from build123d import *

# Parameters (mm, degrees)
SKETCH_4_W      = 37
SKETCH_4_H      = 57
EXTRUDE_1_DEPTH = 2
SKETCH_5_W      = 5.285714285
SKETCH_5_H      = 2
SKETCH_5_W_2    = 5.285714286
EXTRUDE_2_DEPTH = 2
EXTRUDE_START   = -57
SKETCH_5_3_W    = 5.285714285
SKETCH_5_3_H    = 2
SKETCH_5_3_W_2  = 5.285714286
EXTRUDE_3_DEPTH = 2
SKETCH_6_W      = 8.142857143
SKETCH_6_H      = 2
SKETCH_6_W_2    = 8.142857142
EXTRUDE_4_DEPTH = 2
EXTRUDE_START_2 = -37
SKETCH_6_2_W    = 8.142857143
SKETCH_6_2_H    = 2
SKETCH_6_2_W_2  = 8.142857142
EXTRUDE_5_DEPTH = 2


with BuildPart() as part:
    # 草图4 → 凸台-拉伸1 (new body)
    with BuildSketch(Plane(origin=(0, 0, 0), x_dir=(1, 0, 0), z_dir=(0, 1, 0))):
        Rectangle(SKETCH_4_W, SKETCH_4_H)
    extrude(amount=EXTRUDE_1_DEPTH)

    # 草图5 → 凸台-拉伸2 (add)
    with BuildSketch(Plane.XY.offset(28.5)):
        with Locations((10.571428572, 1)):
            Rectangle(SKETCH_5_W, SKETCH_5_H)
        with Locations((0, 1)):
            Rectangle(SKETCH_5_W_2, SKETCH_5_H)
        with Locations((-10.571428572, 1)):
            Rectangle(SKETCH_5_W, SKETCH_5_H)
    extrude(amount=EXTRUDE_2_DEPTH)

    # 草图5<3> → 凸台-拉伸3 (add)
    with BuildSketch(Plane.XY.offset(28.5).offset(EXTRUDE_START)):
        with Locations((10.571428572, 1)):
            Rectangle(SKETCH_5_3_W, SKETCH_5_3_H)
        with Locations((0, 1)):
            Rectangle(SKETCH_5_3_W_2, SKETCH_5_3_H)
        with Locations((-10.571428572, 1)):
            Rectangle(SKETCH_5_3_W, SKETCH_5_3_H)
    extrude(amount=-EXTRUDE_3_DEPTH)

    # 草图6 → 凸台-拉伸4 (add)
    with BuildSketch(Plane(origin=(18.5, 0, 0), x_dir=(0, 0, -1), z_dir=(1, 0, 0))):
        with Locations((-16.285714286, 1)):
            Rectangle(SKETCH_6_W, SKETCH_6_H)
        with Locations((0, 1)):
            Rectangle(SKETCH_6_W_2, SKETCH_6_H)
        with Locations((16.285714286, 1)):
            Rectangle(SKETCH_6_W, SKETCH_6_H)
    extrude(amount=EXTRUDE_4_DEPTH)

    # 草图6<2> → 凸台-拉伸5 (add)
    with BuildSketch(Plane(origin=(18.5, 0, 0), x_dir=(0, 0, -1), z_dir=(1, 0, 0)).offset(EXTRUDE_START_2)):
        with Locations((-16.285714286, 1)):
            Rectangle(SKETCH_6_2_W, SKETCH_6_2_H)
        with Locations((0, 1)):
            Rectangle(SKETCH_6_2_W_2, SKETCH_6_2_H)
        with Locations((16.285714286, 1)):
            Rectangle(SKETCH_6_2_W, SKETCH_6_2_H)
    extrude(amount=-EXTRUDE_5_DEPTH)


solid = part.part
Build history of the part. All positions in model axes, mm. A direction names the side the tool comes from. Give positions to 0.01 mm unless a question says otherwise; leave off trailing zeros. Order: outer loops, then holes, each group sorted by start corner. A loop starts at its lowest first (then second) coordinate and runs counter-clockwise, first axis right, second up. Notation, with made-up numbers: M 62.5,34 L 72.5,34 A14 ccw 72.5,43 Z; hole C 61,85 d7. An arc over 180 degrees is marked long. Use one line per item in the form item = value.
1) Saw through at A-A (x = 16). Give the cut face in (y, z).
Calculated:
outline = M 0,-28.5 L 2,-28.5 L 2,28.5 L 0,28.5 Z
2) Saw through at B-B (z = 8). Give the cut face in (x, y), plus the area to 3 significant figures.
Calculated:
outline = M -18.5,0 L 18.5,0 L 18.5,2 L -18.5,2 Z
area = 74.0 mm2
3) Tool access for faces 1 (the face through (-16, 1, 28.5)), 2 (the face through (16, 1, 28.5)), 3 (the face through (-18.5, 1, -8)), 4 (the face through (18.5, 1, 8)), 5 (the face through (-16, 1, -28.5)): list every direction of +Z, -Z, +X, -X, +Y, -Y with a clear straight run to the whole face (end or side of a thin tool).
Calculated:
face_1 = +Z, -X, +Y, -Y
face_2 = +Z, +X, +Y, -Y
face_3 = -X, +Y, -Y
face_4 = +X, +Y, -Y
face_5 = -Z, -X, +Y, -Y
4) Probe probe 1 along X at (y, z) = (0.4, -23); probe 2 along Z at (x, y) = (6.5, 1.2). List the from-to ranges inside material, lowest first.
Calculated:
probe_1 = -18.5 to 18.5
probe_2 = -28.5 to 28.5
5) Two-plate mould, pull along X, no slides. Class faces 6 (the face through (0, 0, 0)), 7 (the face through (20.5, 1, 0)), 8 (the face through (2.643, 1, -29)), 9 (the face through (-18.5, 1, 8)): released by +X, released by -X, zero draft, split by the parting line, or undercut.
Calculated:
face_6 = zero draft
face_7 = released by +X
face_8 = undercut
face_9 = released by -X
6) Drop flat-ended pins along their axis: pin 1 (0.6 mm diameter, centred on x = 20, y = 1, fed in from -Z); pin 2 (1 mm diameter, centred on x = -19.5, y = 0.5, fed in from +Z); pin 3 (0.6 mm diameter, centred on y = 0.5, z = 29.5, fed in from +X). Give the stop position or say it passes through.
Calculated:
pin_1 = -20.36
pin_2 = 20.36
pin_3 = 13.21
